Geometry check sheet. Reference: the model listing, model coordinates, mm. A direction names the side the tool comes from. Coordinates: 2 decimals unless noted, no trailing zeros. Order: outer loops, then holes, each group sorted by start corner. A loop starts at its lowest first (then second) coordinate and runs counter-clockwise, first axis right, second up. Notation, with made-up numbers: (21.5, 60.25) -> (46.5, 60.25) arc R29 cw to (46.5, 82.25) -> close; hole circle Ø1 at (-6, -22). An arc over 180 degrees is marked (long way). Answer as CSV lines item,"result". Start each with the question number.
from build123d import *

# Parameters (mm, degrees)
EXTRUDE_1_DEPTH      = 20
EXTRUDE_1_DEPTH_BACK = 20
SKETCH_1_R           = 20
SKETCH_2_W           = 281.151719904
SKETCH_2_H           = 265.807540378
EXTRUDE_2_DEPTH      = 100
SKETCH_3_R           = 20
CUT_EXTRUDE_1_DEPTH  = 20


with BuildPart() as part:
    # 草图1 → 凸台-拉伸1 (new, two sides: drawn at the far end of the back side and taken through both)
    with BuildSketch(Plane.XY.offset(-EXTRUDE_1_DEPTH_BACK)):
        with BuildLine():
            Line((0, 40), (-108.026251169, 40))
            Line((-108.026251169, 40), (-108.026251169, -40))
            Line((-108.026251169, -40), (0, -40))
            ThreePointArc((0, -40), (40, 0), (0, 40))
        make_face()
        Circle(SKETCH_1_R, mode=Mode.SUBTRACT)
    extrude(amount=EXTRUDE_1_DEPTH + EXTRUDE_1_DEPTH_BACK)

    # 草图2 → 凸台-拉伸2 (add)
    with BuildSketch(Plane.ZY.offset(108.026251169)):
        Rectangle(SKETCH_2_W, SKETCH_2_H)
    extrude(amount=EXTRUDE_2_DEPTH)

    # 草图3 → 切除-拉伸1 (cut)
    with BuildSketch(Plane.ZY.offset(208.026251169)):
        Circle(SKETCH_3_R)
    extrude(amount=-CUT_EXTRUDE_1_DEPTH, mode=Mode.SUBTRACT)


solid = part.part
Q1. Sectioned sample at B-B, the plane z = 0. Record the cut outline in (x, y).
Q2. Sectioned sample at D-D, the plane z = -58. Record the cut outline in (x, y), then the cut area to 3 significant figures.
Q3. Sectioned sample at C-C, the plane y = -88. Record the cut outline in (x, z).
Q4. Thickness scan on L1, parallel to Y at x = -202, z = 0; L2, parallel to X at y = 99, z = -78.5; L3, parallel to Y at x = -197, z = 11. Record the ranges inside material, lowest first.
Q5. Sectioned sample at A-A, the plane y = 0. Record the cut outline in (x, z), then the cut area to 3 significant figures.
Q6. Go/stop test with flat-tipped pins: pin 1 Ø20 at (x, z) = (-37.5, 4) entering from +Y; pin 2 Ø10 at (y, z) = (-55, -104) entering from +X; pin 3 Ø12 at (y, z) = (3, 4.5) entering from -X. Record where each tip stops, or that it passes through.
Q7. Release check for a two-part mould opening along Y. For faces 1 (the flat face through (-108.026, 2, 29)), 2 (the cylindrical face through (-4.336, -19.524, -0.28)), 3 (the flat face through (-55, -40, 0)) record: released by +Y, released by -Y, zero draft, split by the parting line, or undercut.
Q8. Access from +Z, -Z, +X, -X, +Y, -Y to the whole of each face (thin tool, end or side, straight path). Record for faces 4 (the flat face through (-51, 1, -20)), 5 (the flat face through (-51, 1, 20)), 6 (the flat face through (-53, 40, 0)), 7 (the cylindrical face through (-198.166, -19.524, -4.336)), 8 (the cylindrical face through (39.99, -0.88, -0.28)).
Geometry results:
1,outline,"(-208.03, -132.9) -> (-108.03, -132.9) -> (-108.03, -40) -> (0, -40) arc R40 ccw to (0, 40) -> (-108.03, 40) -> (-108.03, 132.9) -> (-208.03, 132.9) -> (-208.03, 20) -> (-188.03, 20) -> (-188.03, -20) -> (-208.03, -20) -> close; hole circle Ø40 at (0, 0)"
2,outline,"(-208.03, -132.9) -> (-108.03, -132.9) -> (-108.03, 132.9) -> (-208.03, 132.9) -> close"
2,area,"26,600 mm^2"
3,outline,"(-208.03, -140.58) -> (-108.03, -140.58) -> (-108.03, 140.58) -> (-208.03, 140.58) -> close"
4,L1,"y = -132.9 to -20, 20 to 132.9"
4,L2,"x = -208.03 to -108.03"
4,L3,"y = -132.9 to -16.7, 16.7 to 132.9"
5,outline,"(-208.03, -140.58) -> (-108.03, -140.58) -> (-108.03, -20) -> (-20, -20) -> (-20, 20) -> (-108.03, 20) -> (-108.03, 140.58) -> (-208.03, 140.58) -> (-208.03, 20) -> (-188.03, 20) -> (-188.03, -20) -> (-208.03, -20) -> close; (20, -20) -> (40, -20) -> (40, 20) -> (20, 20) -> close"
5,area,"31,600 mm^2"
6,pin 1,"stops at y = 40"
6,pin 2,"stops at x = -108.03"
6,pin 3,"stops at x = -188.03"
7,face 1,"zero draft"
7,face 2,"undercut"
7,face 3,"released by -Y"
8,face 4,"-Z, +X, +Y, -Y"
8,face 5,"+Z, +X, +Y, -Y"
8,face 6,"+Z, -Z, +X, +Y"
8,face 7,"-X"
8,face 8,"+Z, -Z, +X"
